from build123d import *

# Parameters (mm, degrees)
SKETCH1_R           = 1.450000006
SKETCH1_R_2         = 1.45
SKETCH1_R_3         = 38
SKETCH1_W           = 6.2
SKETCH1_H           = 3.4
BOSS_EXTRUDE1_DEPTH = 5.85


with BuildPart() as part:
    # Sketch1 → Boss-Extrude1 (new body)
    with BuildSketch(Plane.XY):
        with BuildLine():
            Line((587.995290395, 497.753361998), (601.026388312, 465.269666287))
            ThreePointArc((601.026388312, 465.269666287), (600.580353033, 449.003385667), (588.406365105, 438.205939183))
            Line((588.406365105, 438.205939183), (555.146182231, 427.30822221))
            ThreePointArc((555.146182231, 427.30822221), (551.939243509, 422.882775531), (555.146182231, 418.457328853))
            Line((555.146182231, 418.457328853), (588.406366938, 407.55961128))
            ThreePointArc((588.406366938, 407.55961128), (600.58035448, 396.762164902), (601.026389221, 380.495884628))
            Line((601.026389221, 380.495884628), (587.995289899, 348.01218948))
            ThreePointArc((587.995289899, 348.01218948), (589.32399836, 342.710908714), (594.775468563, 342.322944064))
            Line((594.775468563, 342.322944064), (633.210915705, 366.208380082))
            ThreePointArc((633.210915705, 366.208380082), (644.436635852, 371.181514399), (656.596182238, 372.882775531))
            ThreePointArc((656.596182238, 372.882775531), (668.755728624, 371.181514399), (679.981448771, 366.208380082))
            Line((679.981448771, 366.208380082), (718.416895913, 342.322944064))
            ThreePointArc((718.416895913, 342.322944064), (723.868366115, 342.710908714), (725.197074576, 348.01218948))
            Line((725.197074576, 348.01218948), (712.165975255, 380.495884628))
            ThreePointArc((712.165975255, 380.495884628), (712.612009996, 396.762164902), (724.785997538, 407.559611279))
            Line((724.785997538, 407.559611279), (758.046182244, 418.457328853))
            ThreePointArc((758.046182244, 418.457328853), (761.253120966, 422.882775531), (758.046182244, 427.30822221))
            Line((758.046182244, 427.30822221), (724.785999371, 438.205939183))
            ThreePointArc((724.785999371, 438.205939183), (712.612011443, 449.003385667), (712.165976164, 465.269666287))
            Line((712.165976164, 465.269666287), (725.197074081, 497.753361998))
            ThreePointArc((725.197074081, 497.753361998), (723.86836572, 503.054641878), (718.416896408, 503.442606583))
            Line((718.416896408, 503.442606583), (679.981448771, 479.557172561))
            ThreePointArc((679.981448771, 479.557172561), (668.755728555, 474.584038083), (656.596182238, 472.882775531))
            ThreePointArc((656.596182238, 472.882775531), (644.436635921, 474.584038083), (633.210915705, 479.557172561))
            Line((633.210915705, 479.557172561), (594.775468067, 503.442606583))
            ThreePointArc((594.775468067, 503.442606583), (589.323998755, 503.054641878), (587.995290395, 497.753361998))
        make_face()
        with Locations((592.317421269, 499.487219843)):
            Circle(SKETCH1_R, mode=Mode.SUBTRACT)
        with Locations(Location((706.596182238, 432.882775531, 0), (0, 0, 180))):
            Circle(SKETCH1_R_2, mode=Mode.SUBTRACT)
        with Locations(Location((706.596182238, 442.882775531, 0), (0, 0, 180))):
            Circle(SKETCH1_R_2, mode=Mode.SUBTRACT)
        with Locations(Location((706.596182238, 452.882775531, 0), (0, 0, 180))):
            Circle(SKETCH1_R_2, mode=Mode.SUBTRACT)
        with Locations((706.596182238, 392.882775531)):
            Circle(SKETCH1_R_2, mode=Mode.SUBTRACT)
        with Locations((556.596182238, 422.882775531)):
            Circle(SKETCH1_R, mode=Mode.SUBTRACT)
        with Locations(Location((646.596182238, 378.882775531, 0), (0, 0, 180))):
            Circle(SKETCH1_R_2, mode=Mode.SUBTRACT)
        with Locations((656.596182238, 422.882775531)):
            Circle(SKETCH1_R_3, mode=Mode.SUBTRACT)
        with Locations(Location((636.596182238, 378.882775531, 0), (0, 0, 180))):
            Circle(SKETCH1_R_2, mode=Mode.SUBTRACT)
        with Locations((706.596182238, 402.882775531)):
            Circle(SKETCH1_R_2, mode=Mode.SUBTRACT)
        with Locations((656.596182238, 466.882775531)):
            Circle(SKETCH1_R_2, mode=Mode.SUBTRACT)
        with Locations((592.317421269, 346.278331219)):
            Circle(SKETCH1_R, mode=Mode.SUBTRACT)
        with Locations((706.596182238, 412.882775531)):
            Circle(SKETCH1_R_2, mode=Mode.SUBTRACT)
        with Locations(Location((656.596182238, 378.882775531, 0), (0, 0, 180))):
            Circle(SKETCH1_R_2, mode=Mode.SUBTRACT)
        with Locations(Location((698.596182238, 442.882775531, 0), (0, 0, 180))):
            Circle(SKETCH1_R_2, mode=Mode.SUBTRACT)
        with Locations((698.596182238, 402.882775531)):
            Circle(SKETCH1_R_2, mode=Mode.SUBTRACT)
        with Locations((646.596182238, 466.882775531)):
            Circle(SKETCH1_R_2, mode=Mode.SUBTRACT)
        with Locations((636.596182238, 466.882775531)):
            Circle(SKETCH1_R_2, mode=Mode.SUBTRACT)
        with Locations(Location((676.596182238, 466.882775531, 0), (0, 0, 180))):
            Circle(SKETCH1_R_2, mode=Mode.SUBTRACT)
        with Locations(Location((666.596182238, 466.882775531, 0), (0, 0, 180))):
            Circle(SKETCH1_R_2, mode=Mode.SUBTRACT)
        with Locations(Location((706.596182238, 422.882775531, 0), (0, 0, 180))):
            Circle(SKETCH1_R_2, mode=Mode.SUBTRACT)
        with Locations(Location((688.596182238, 452.882775531, 0), (0, 0, 180))):
            Circle(SKETCH1_R_2, mode=Mode.SUBTRACT)
        with Locations((688.596182238, 392.882775531)):
            Circle(SKETCH1_R_2, mode=Mode.SUBTRACT)
        with Locations(Location((624.596182238, 392.882775531, 0), (0, 0, 180))):
            Circle(SKETCH1_R_2, mode=Mode.SUBTRACT)
        with Locations(Location((720.874943207, 346.278331219, 0), (0, 0, 180))):
            Circle(SKETCH1_R, mode=Mode.SUBTRACT)
        with Locations((676.596182238, 378.882775531)):
            Circle(SKETCH1_R_2, mode=Mode.SUBTRACT)
        with Locations((666.596182238, 378.882775531)):
            Circle(SKETCH1_R_2, mode=Mode.SUBTRACT)
        with Locations(Location((756.596182238, 422.882775531, 0), (0, 0, 180))):
            Circle(SKETCH1_R, mode=Mode.SUBTRACT)
        with Locations((624.596182238, 452.882775531)):
            Circle(SKETCH1_R_2, mode=Mode.SUBTRACT)
        with Locations((606.596182238, 422.882775531)):
            Circle(SKETCH1_R_2, mode=Mode.SUBTRACT)
        with Locations(Location((720.874943207, 499.487219843, 0), (0, 0, 180))):
            Circle(SKETCH1_R, mode=Mode.SUBTRACT)
        with Locations(Location((614.596182238, 402.882775531, 0), (0, 0, 180))):
            Circle(SKETCH1_R_2, mode=Mode.SUBTRACT)
        with Locations((614.596182238, 442.882775531)):
            Circle(SKETCH1_R_2, mode=Mode.SUBTRACT)
        with Locations(Location((606.596182238, 412.882775531, 0), (0, 0, 180))):
            Circle(SKETCH1_R_2, mode=Mode.SUBTRACT)
        with Locations(Location((606.596182238, 402.882775531, 0), (0, 0, 180))):
            Circle(SKETCH1_R_2, mode=Mode.SUBTRACT)
        with Locations(Location((606.596182238, 392.882775531, 0), (0, 0, 180))):
            Circle(SKETCH1_R_2, mode=Mode.SUBTRACT)
        with Locations((606.596182238, 452.882775531)):
            Circle(SKETCH1_R_2, mode=Mode.SUBTRACT)
        with Locations((606.596182238, 442.882775531)):
            Circle(SKETCH1_R_2, mode=Mode.SUBTRACT)
        with Locations((606.596182238, 432.882775531)):
            Circle(SKETCH1_R_2, mode=Mode.SUBTRACT)
        with BuildLine():
            Line((594.852213644, 494.089955534), (608.369257372, 460.394902501))
            ThreePointArc((608.369257372, 460.394902501), (609.936297881, 459.027594122), (611.962982661, 459.494174197))
            Line((611.962982661, 459.494174197), (628.291466753, 473.195399177))
            ThreePointArc((628.291466753, 473.195399177), (629.102888547, 475.11027328), (628.028466383, 476.890937531))
            Line((628.028466383, 476.890937531), (597.192526929, 496.053711548))
            ThreePointArc((597.192526929, 496.053711548), (595.310843783, 495.919797808), (594.852213644, 494.089955534))
        make_face(mode=Mode.SUBTRACT)
        with Locations((698.596182238, 392.882775531)):
            Rectangle(SKETCH1_W, SKETCH1_H, mode=Mode.SUBTRACT)
        with BuildLine():
            Line((562.360059701, 421.35524452), (599.360059701, 409.232174436))
            ThreePointArc((599.360059701, 409.232174436), (601.41475291, 409.553708225), (602.360059701, 411.406150729))
            Line((602.360059701, 411.406150729), (602.360059701, 434.359400333))
            ThreePointArc((602.360059701, 434.359400333), (601.41475291, 436.211842837), (599.360059701, 436.533376627))
            Line((599.360059701, 436.533376627), (562.360059701, 424.410306542))
            ThreePointArc((562.360059701, 424.410306542), (561.253120966, 422.882775531), (562.360059701, 421.35524452))
        make_face(mode=Mode.SUBTRACT)
        with BuildLine():
            Line((594.85221424, 351.675595364), (608.369259134, 385.370647084))
            ThreePointArc((608.369259134, 385.370647084), (609.936299703, 386.737955426), (611.962984497, 386.271375324))
            Line((611.962984497, 386.271375324), (628.291464916, 372.570153427))
            ThreePointArc((628.291464916, 372.570153427), (629.102886739, 370.655279313), (628.028464622, 368.874615009))
            Line((628.028464622, 368.874615009), (597.192526664, 349.711840073))
            ThreePointArc((597.192526664, 349.711840073), (595.310844178, 349.845753725), (594.85221424, 351.675595364))
        make_face(mode=Mode.SUBTRACT)
        with Locations((614.596182238, 452.882775531)):
            Rectangle(SKETCH1_W, SKETCH1_H, mode=Mode.SUBTRACT)
        with Locations((698.596182238, 452.882775531)):
            Rectangle(SKETCH1_W, SKETCH1_H, mode=Mode.SUBTRACT)
        with BuildLine():
            Line((715.999837812, 349.711840073), (685.163899854, 368.874615009))
            ThreePointArc((685.163899854, 368.874615009), (684.089477737, 370.655279313), (684.900899559, 372.570153427))
            Line((684.900899559, 372.570153427), (701.229379978, 386.271375324))
            ThreePointArc((701.229379978, 386.271375324), (703.256064773, 386.737955426), (704.823105342, 385.370647084))
            Line((704.823105342, 385.370647084), (718.340150235, 351.675595364))
            ThreePointArc((718.340150235, 351.675595364), (717.881520298, 349.845753725), (715.999837812, 349.711840073))
        make_face(mode=Mode.SUBTRACT)
        with BuildLine():
            Line((750.832304774, 424.410306542), (713.832304774, 436.533376627))
            ThreePointArc((713.832304774, 436.533376627), (711.777611566, 436.211842837), (710.832304774, 434.359400333))
            Line((710.832304774, 434.359400333), (710.832304774, 411.406150729))
            ThreePointArc((710.832304774, 411.406150729), (711.777611565, 409.553708225), (713.832304774, 409.232174436))
            Line((713.832304774, 409.232174436), (750.832304774, 421.35524452))
            ThreePointArc((750.832304774, 421.35524452), (751.939243509, 422.882775531), (750.832304774, 424.410306542))
        make_face(mode=Mode.SUBTRACT)
        with BuildLine():
            Line((684.900897722, 473.195399177), (701.229381815, 459.494174197))
            ThreePointArc((701.229381815, 459.494174197), (703.256066594, 459.027594122), (704.823107103, 460.394902501))
            Line((704.823107103, 460.394902501), (718.340150832, 494.089955534))
            ThreePointArc((718.340150832, 494.089955534), (717.881520693, 495.919797808), (715.999837547, 496.053711548))
            Line((715.999837547, 496.053711548), (685.163898093, 476.890937531))
            ThreePointArc((685.163898093, 476.890937531), (684.089475929, 475.11027328), (684.900897722, 473.195399177))
        make_face(mode=Mode.SUBTRACT)
        with Locations((614.596182238, 392.882775531)):
            Rectangle(SKETCH1_W, SKETCH1_H, mode=Mode.SUBTRACT)
    extrude(amount=BOSS_EXTRUDE1_DEPTH)


solid = part.part
Part model, mm, in its own coordinate system. A direction names the side the tool comes from. Coordinates: 2 decimals unless noted, no trailing zeros. Order: outer loops, then holes, each group sorted by start corner. A loop starts at its lowest first (then second) coordinate and runs counter-clockwise, first axis right, second up. Notation, with made-up numbers: M 26,39.5 L 65,39.5 A18 ccw 65,55.5 Z; hole C -8,42 d8. An arc over 180 degrees is marked long. Use a Markdown table: item, result.
(1) Pull direction X, two halves, no side cores. Call faces 1 (the flat face through (695, 423, 5.85)), 2 (the flat face through (580.6, 415.38, 2.88)), 3 (the flat face through (571.5, 413.1, 2.9)): released by +X, released by -X, zero draft, split by the parting line, or undercut.
A:
| item | result |
|---|---|
| face 1 | zero draft |
| face 2 | undercut |
| face 3 | released by -X |
(2) Cut at B-B on y = 363. Write the cut outline in (x, z), then the cut area to 3 significant figures.
A:
| item | result |
|---|---|
| outline | M 594.01,0 L 599.4,0 L 599.4,5.85 L 594.01,5.85 Z; M 618.58,0 L 628.05,0 L 628.05,5.85 L 618.58,5.85 Z; M 685.14,0 L 694.62,0 L 694.62,5.85 L 685.14,5.85 Z; M 713.8,0 L 719.18,0 L 719.18,5.85 L 713.8,5.85 Z |
| area | 174 mm^2 |
(3) Cut at D-D on z = 4.5. State how many separate pieces and enclosed holes the cut face has, then the cut area to 3 significant figures.
A:
| item | result |
|---|---|
| separate pieces | 1 |
| enclosed holes | 49 |
| area | 8,390 mm^2 |
(4) Probe L1, parallel to Y at x = 656.5, z = 3.1; L2, parallel to X at y = 368, z = 0.35; L3, parallel to X at y = 377, z = 4.85. List the from-to ranges inside material, lowest first.
A:
| item | result |
|---|---|
| L1 | y = 372.88 to 377.44, 380.33 to 384.88, 460.88 to 465.44, 468.33 to 472.88 |
| L2 | x = 596.01 to 601.4, 626.62 to 636.38, 676.82 to 686.57, 711.79 to 717.18 |
| L3 | x = 599.62 to 605.01, 623.01 to 690.18, 708.18 to 713.57 |
(5) Cut at A-A on x = 734.5. Write the cut outline in (y, z).
A:
| item | result |
|---|---|
| outline | M 410.74,0 L 416,0 L 416,5.85 L 410.74,5.85 Z; M 429.76,0 L 435.02,0 L 435.02,5.85 L 429.76,5.85 Z |
(6) Tool access for faces 4 (the flat face through (620.013, 466.249, 2.884)), 5 (the flat face through (594.6, 364.48, 2.88)), 6 (the flat face through (699.47, 491.67, 2.88)), 7 (the flat face through (613.724, 354.098, 2.884)): list every direction of +Z, -Z, +X, -X, +Y, -Y with a clear straight run to the whole face (end or side of a thin tool).
A:
| item | result |
|---|---|
| face 4 | +Z, -Z |
| face 5 | +Z, -Z, -X |
| face 6 | +Z, -Z, +Y |
| face 7 | +Z, -Z, -Y |
(7) Cut at C-C on x = 641.5. Write the cut outline in (y, z), then the cut area to 3 significant figures.
A:
| item | result |
|---|---|
| outline | M 370.23,0 L 388.01,0 L 388.01,5.85 L 370.23,5.85 Z; M 457.76,0 L 475.53,0 L 475.53,5.85 L 457.76,5.85 Z |
| area | 208 mm^2 |
(8) Flat gauge pins, fed straight in: pin 1 (3.5 mm diameter, centred on x = 606.6, y = 432.88, fed in from -Z); pin 2 (2.5 mm diameter, centred on y = 393, z = 2.5, fed in from +X); pin 3 (1.5 mm diameter, centred on y = 472.5, z = 2, fed in from -X) (3 decimals); pin 4 (1 mm diameter, centred on x = 643, z = 4.5, fed in from -Y). Where does each tip first touch, or does it go through?
A:
| item | result |
|---|---|
| pin 1 | stops at z = 0 |
| pin 2 | stops at x = 711.64 |
| pin 3 | stops at x = 597.825 |
| pin 4 | stops at y = 370.58 |
